CAD build for the part. Positions are in the model's coordinates, mm. A direction names the side the tool comes from. Give positions to 0.01 mm unless a question says otherwise; leave off trailing zeros. Write each loop counter-clockwise with the first axis right and the second up, starting at its lowest first coordinate (ties: lowest second). Pieces come first, ordered by that corner, then holes. Notation, with made-up numbers: M 10.25,23.5 L 64.25,23.5 A17 cw 64.25,34.5 Z; hole C -9.5,34.5 d1. An arc over 180 degrees is marked long. One line per question, with ' | ' between items. Start each with the question number.
1. Cut at A-A, the plane y = 7.5. Write the cut outline in (x, z) (3 decimals).
2. Flat gauge pins, fed straight in: pin 1 (0.9 mm diameter, centred on x = -39, z = -19, fed in from +Y); pin 2 (6.5 mm diameter, centred on x = -73, z = -26, fed in from +Y) (3 decimals). Where does each tip first touch, or does it go through?
3. Wall check: L1, parallel to X at y = 8.5, z = -32.5; L2, parallel to X at y = 2.25, z = -22.75; L3, parallel to X at y = 12.75, z = -25. Give the ranges that are in metal, low to high.
4. Pull direction X, two halves, no side cores. Call faces 1 (the face through (-38, 0, -23)), 2 (the face through (8.372, 7, -23)), 3 (the face through (-2.86, 4.83, -20.38)): released by +X, released by -X, zero draft, split by the parting line, or undercut.
5. Cut at D-D, the plane y = 1.75. Write the cut outline in (x, z) (3 decimals), then the cut area to 3 significant figures.
6. Which spindle directions (+Z, -Z, +X, -X, +Y, -Y) get a long thin tool onto all of the face, cutting with end or side? Do faces 4 (the face through (-14, 14.288, -23)), 5 (the face through (-36.935, 8, -23)), 6 (the face through (-5.704, 11.94, -16.996)). Say none if no direction does.
7. Cut at B-B, the plane z = -15.5. Write the cut outline in (x, y), then the cut area to 3 significant figures.
8. Cut at C-C, the plane x = -4.5. Write the cut outline in (y, z) (1 decimal), then the cut area to 3 significant figures.
Autodesk Inventor part; units mm, degrees
ref_plane "YZ Plane" through (0, 0, 0) normal (1, 0, 0) x (0, 1, 0)
ref_plane "XZ Plane" through (0, 0, 0) normal (0, 1, 0) x (-1, 0, 0)
ref_plane "XY Plane" through (0, 0, 0) normal (0, 0, 1) x (1, 0, 0)
sketch "Sketch1" plane through (0, 0, 0) normal (0, 1, 0) x (-1, 0, 0)
  line L0 (85.2904, -33.5134) -> (-8.3721, -33.5134)
  line L1 (-8.3721, -33.5134) -> (-8.3721, -12.8759)
  line L2 (-8.3721, -12.8759) -> (85.2904, -12.8759)
  line L3 (85.2904, -12.8759) -> (85.2904, -33.5134)
  point P0 (0, 0)
  dimension "d0" = 93.6625
  dimension "d1" = 20.6375
extrude "Extrusion1" add sketch "Sketch1" along normal blind 14.2875
sketch "Sketch2" plane through (0, 14.2875, 0) normal (0, 1, 0) x (1, 0, 0)
  line L0 (8.3721, 33.5134) -> (-85.2904, 33.5134)
  line L1 (-85.2904, 33.5134) -> (-85.2904, 12.8759)
  line L2 (-85.2904, 12.8759) -> (8.3721, 12.8759)
  line L3 (8.3721, 12.8759) -> (8.3721, 33.5134)
  line L4 (-85.2904, 23.1947) -> (8.3721, 23.1947) construction
  line L5 (-4.3279, 33.5134) -> (-4.3279, 12.8759) construction
  line L6 (-72.5904, 33.5134) -> (-72.5904, 12.8759) construction
  circle A0 centre (-72.5904, 23.1947) radius 3.175
  circle A1 centre (-4.3279, 23.1947) radius 3.175
  point P0 (0, 0)
  dimension "d4" = 12.7
  dimension "d5" = 12.7
  dimension "d6" = 6.35
  dimension "d7" = 6.35
extrude "Extrusion2" cut sketch "Sketch2" against normal blind 14.2875 contours A0 | A1
sketch "Sketch3" plane through (0, 14.2875, 0) normal (0, 1, 0) x (1, 0, 0)
  circle A0 centre (-72.5904, 23.1947) radius 3.175
  circle A1 centre (-4.3279, 23.1947) radius 3.175
  circle A2 centre (-72.5904, 23.1947) radius 6.35
  circle A3 centre (-4.3279, 23.1947) radius 6.35
  point P0 (0, 0)
  point P1 (8.3721, 33.5134)
  point P2 (-85.2904, 33.5134)
  dimension "d10" = 12.7
  dimension "d11" = 12.7
  dimension "d14" = 68.2625
  dimension "d16" = 93.6625
extrude "Extrusion3" cut sketch "Sketch3" against normal blind 4.7625
sketch "Sketch4" plane through (0, 14.2875, 0) normal (0, 1, 0) x (1, 0, 0)
  line L0 (8.3721, 33.5134) -> (-85.2904, 33.5134)
  line L1 (-85.2904, 12.8759) -> (8.3721, 12.8759)
  line L2 (-38.4591, 33.5134) -> (-38.4591, 12.8759) construction
  line L3 (-38.4591, 23.1947) -> (-36.9351, 23.1947) construction
  line L4 (-36.9351, 23.1947) -> (-39.9831, 23.1947) construction
  line L5 (-39.9831, 33.5134) -> (-39.9831, 12.8759)
  line L6 (-39.9831, 12.8759) -> (-36.9351, 12.8759)
  line L7 (-36.9351, 12.8759) -> (-36.9351, 33.5134)
  line L8 (-39.9831, 33.5134) -> (-36.9351, 33.5134)
  point P0 (0, 0)
  dimension "d19" = 1.524
  dimension "d21" = 3.048
extrude "Extrusion4" cut sketch "Sketch4" against normal blind 11.7602
equation "\"d5\" = d4"
equation "\"d6\" = d7"
equation "\"d10\" = d11"
properties part number "Battery Base"
Here are the results:
1) outline: M -85.29,-33.513 L -39.983,-33.513 L -39.983,-12.876 L -85.29,-12.876 Z; M -36.935,-33.513 L 8.372,-33.513 L 8.372,-12.876 L -36.935,-12.876 Z; hole C -72.59,-23.195 d6.35; hole C -4.328,-23.195 d6.35
2) pin 1: y = 2.53 | pin 2: y = 9.525
3) L1: -85.29 to -39.98, -36.94 to 8.37 | L2: -85.29 to -75.73, -69.45 to -7.47, -1.18 to 8.37 | L3: -85.29 to -78.68, -66.5 to -39.98, -36.94 to -10.42, 1.76 to 8.37
4) face 1: zero draft | face 2: released by +X | face 3: undercut
5) outline: M -85.29,-33.513 L 8.372,-33.513 L 8.372,-12.876 L -85.29,-12.876 Z; hole C -72.59,-23.195 d6.35; hole C -4.328,-23.195 d6.35 | area: 1,870 mm^2
6) face 4: +Z, -Z, +X, -X, +Y | face 5: +Z, -Z, +Y | face 6: +Y
7) outline: M -85.29,0 L 8.37,0 L 8.37,14.29 L -36.94,14.29 L -36.94,2.53 L -39.98,2.53 L -39.98,14.29 L -85.29,14.29 Z | area: 1,300 mm^2
8) outline: M 0,-33.5 L 14.3,-33.5 L 14.3,-29.5 L 9.5,-29.5 L 9.5,-26.4 L 0,-26.4 Z; M 0,-20 L 9.5,-20 L 9.5,-16.8 L 14.3,-16.8 L 14.3,-12.9 L 0,-12.9 Z | area: 174 mm^2
